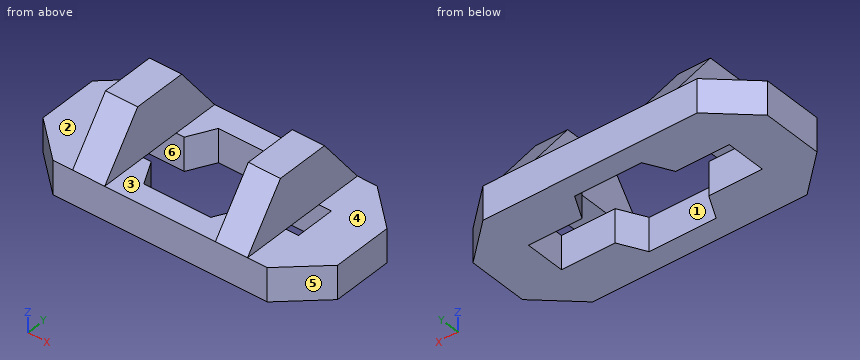
```python
from build123d import *

# Parameters (mm, degrees)
EXTRUDE1_DEPTH = 25


with BuildPart() as part:
    # Sketch1 → Extrude1 (new body)
    with BuildSketch(Plane.XY):
        Polygon((110, 22.5), (110, -22.5), (80, -50), (-80, -50), (-110, -22.5), (-110, 22.5), (-80, 50), (80, 50), align=None)
        Polygon((-75.325078699, 15), (-35.325078699, 15), (-25.325078699, 33.914218403), (24.674921301, 33.914218403), (34.674921301, 15), (74.674921301, 15), (74.674921301, -15), (34.674921301, -15), (24.674921301, -33.914218403), (-25.325078699, -33.914218403), (-35.325078699, -15), (-75.325078699, -15), align=None, mode=Mode.SUBTRACT)
    extrude(amount=EXTRUDE1_DEPTH)

    # Sketch3 → Loft1 section 0
    with BuildSketch(Plane.XY.offset(25)):
        with BuildLine():
            Line((-65.325078699, -50), (-41.325078699, -50))
            Line((-41.325078699, -50), (-41.325078699, 50))
            Line((-41.325078699, 50), (-65.325078699, 50))
            Line((-65.325078699, 50), (-65.325078699, -50))
        make_face()
    # Sketch2 → Loft1 section 1
    with BuildSketch(Plane.XY.offset(65)):
        with BuildLine():
            Line((-65.325078699, 20), (-41.325078699, 20))
            Line((-41.325078699, 20), (-41.325078699, -20))
            Line((-41.325078699, -20), (-65.325078699, -20))
            Line((-65.325078699, -20), (-65.325078699, 20))
        make_face()
    loft1 = loft()

    # Mirror1: Loft1 across plane
    add(loft1.mirror(Plane(origin=(0, 0, 0), x_dir=(0, 0, 1), z_dir=(1, 0, 0))))


solid = part.part
```
Design review of the part built by this model. Coordinates are the model's own, in mm. Face numbers are marked on the shaded views. A direction names the side the tool comes from. Give positions to 0.01 mm unless a question says otherwise; leave off trailing zeros. Write each loop counter-clockwise with the first axis right and the second up, starting at its lowest first coordinate (ties: lowest second). Pieces come first, ordered by that corner, then holes.
(1) Wall thickness on line 1 along X through (y, z) = (-6.5, 6.5); line 2 along X through (y, z) = (31.5, 29); line 3 along Y through (x, z) = (-24, 24): over which ranges is each line inside the solid? List them lowest first.
Checked values:
line 1: x = -110 to -75.33, 74.67 to 110
line 2: x = -65.33 to -41.33, 41.33 to 65.33
line 3: y = -50 to -33.91, 33.91 to 50
(2) Add section B-B (z = 11). Give the boundary of the cut face in (x, y), and give its area (3 significant figures).
Checked values:
outline: (-110, -22.5) - (-80, -50) - (80, -50) - (110, -22.5) - (110, 22.5) - (80, 50) - (-80, 50) - (-110, 22.5) - close; hole (-75.33, -15) - (-35.33, -15) - (-25.33, -33.91) - (24.67, -33.91) - (34.67, -15) - (74.67, -15) - (74.67, 15) - (34.67, 15) - (24.67, 33.91) - (-25.33, 33.91) - (-35.33, 15) - (-75.33, 15) - close
area: 13,600 mm2
(3) Mouldability with a two-part tool opening along X and no side actions: class the marked faces 4, 5 and 6 as +X half, -X half, draft (parallel to the pull), parting line (faces both ways), or undercut.
Checked values:
face 4: draft
face 5: +X half
face 6: undercut
(4) Tool access review of the marked faces 1, 2 and 3: name each direction out of +Z, -Z, +X, -X, +Y, -Y from which nothing blocks a thin tool from reaching the whole face with its end or side.
Checked values:
face 1: +Z, -Z
face 2: +Z, -X, +Y, -Y
face 3: +Z, +Y, -Y
(5) Add section A-A (x = -11.5). Give the boundary of the cut face in (y, z), and give its area (3 significant figures).
Checked values:
outline: (-50, 0) - (-33.91, 0) - (-33.91, 25) - (-50, 25) - close; (33.91, 0) - (50, 0) - (50, 25) - (33.91, 25) - close
area: 804 mm2
(6) Clearance check with flat-ended pins moving along their axes: pin 1 Ø8 at (y, z) = (32, 58) entering from -X; pin 2 Ø5 at (y, z) = (13.5, 40.5) entering from -X; pin 3 Ø7 at (x, y) = (-57.5, 7) entering from -Z; pin 4 Ø10.5 at (x, y) = (19.5, 40.5) entering from +Z. State where each tip first meets the part, or that it passes through.
Checked values:
pin 1: passes through
pin 2: stops at x = -65.33
pin 3: stops at z = 25
pin 4: stops at z = 25
(7) Add section C-C (y = 10). Give the number of separate pieces and of enclosed holes in the cut face, and give its area (3 significant figures).
Checked values:
separate pieces: 4
enclosed holes: 0
area: 3,670 mm2
(8) Add section D-D (x = -61.5). Give the boundary of the cut face in (y, z).
Checked values:
outline: (-50, 0) - (-15, 0) - (-15, 25) - (15, 25) - (15, 0) - (50, 0) - (50, 25) - (20, 65) - (-20, 65) - (-50, 25) - close
